Input: part model. Units: mm. Frame: model coordinates. Round coordinates to 2 decimals unless told otherwise and drop trailing zeros. Write each question's results on one line, items separated by ' | '.
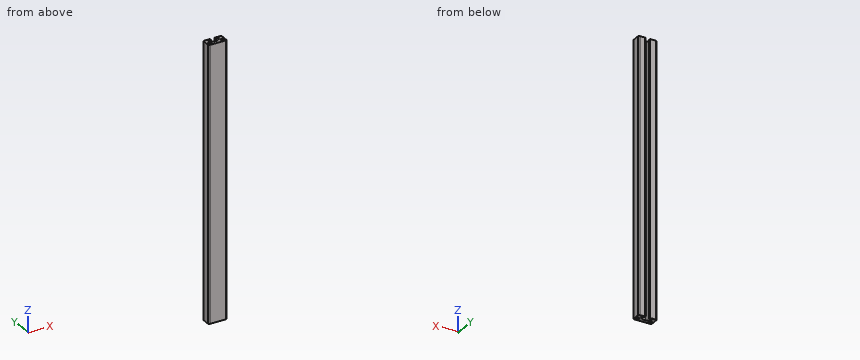
from build123d import *

# Parameters (mm, degrees)
SKETCH3_R           = 2.1463
BOSS_EXTRUDE1_DEPTH = 190.5
FILLET1_R           = 0.254


with BuildPart() as part:
    # Sketch3 → Boss-Extrude1 (new body, symmetric)
    with BuildSketch(Plane.XY):
        with BuildLine():
            Line((-11.049, 12.7), (-3.302, 12.7))
            Line((-3.302, 12.7), (-3.302, 10.328863887))
            Line((-3.302, 10.328863887), (-6.985, 10.328863887))
            ThreePointArc((-6.985, 10.328863887), (-7.454330803, 10.01526707), (-7.344210245, 9.461653642))
            Line((-7.344210245, 9.461653642), (-3.452505379, 5.569948776))
            ThreePointArc((-3.452505379, 5.569948776), (-2.628470073, 5.019345987), (-1.656454155, 4.826))
            Line((-1.656454155, 4.826), (1.656454155, 4.826))
            ThreePointArc((1.656454155, 4.826), (2.628470073, 5.019345987), (3.452505379, 5.569948776))
            Line((3.452505379, 5.569948776), (7.344210245, 9.461653642))
            ThreePointArc((7.344210245, 9.461653642), (7.454330803, 10.01526707), (6.985, 10.328863887))
            Line((6.985, 10.328863887), (3.302, 10.328863887))
            Line((3.302, 10.328863887), (3.302, 12.7))
            Line((3.302, 12.7), (11.049, 12.7))
            ThreePointArc((11.049, 12.7), (12.216433296, 12.216433296), (12.7, 11.049))
            Line((12.7, 11.049), (12.7, 1.651))
            ThreePointArc((12.7, 1.651), (12.216433296, 0.483566704), (11.049, 0))
            Line((11.049, 0), (-11.049, 0))
            ThreePointArc((-11.049, 0), (-12.216433296, 0.483566704), (-12.7, 1.651))
            Line((-12.7, 1.651), (-12.7, 11.049))
            ThreePointArc((-12.7, 11.049), (-12.216433296, 12.216433296), (-11.049, 12.7))
        make_face()
        with Locations((8.509, 4.064)):
            Circle(SKETCH3_R, mode=Mode.SUBTRACT)
        with Locations((-8.509, 4.064)):
            Circle(SKETCH3_R, mode=Mode.SUBTRACT)
    extrude(amount=BOSS_EXTRUDE1_DEPTH, both=True)

    # Fillet1
    fillet1_edges = [part.edges().sort_by_distance(p)[0] for p in [
        (-3.302, 12.7, 0),
        (-3.302, 10.328863887, 0),
        (3.302, 10.328863887, 0),
        (3.302, 12.7, 0),
    ]]
    fillet(fillet1_edges, radius=FILLET1_R)


solid = part.part
1. Section query A-A, the plane z = 158.5. Count the separate pieces of the cut face and the enclosed holes in it, plus the area to 3 significant figures.
Answer:
separate pieces: 1 | enclosed holes: 2 | area: 216 mm^2
2. Contact query for a flat-ended pin moving along its axis: pin 1 (3.5 mm diameter, centred on x = -0.5, z = -2.5, fed in from +Y). Output: stop coordinate, or through.
Answer:
pin 1: y = 4.9
3. Line query: line 1 (X direction, y = 11, z = 91); line 2 (Y direction, x = 3.5, z = -4); line 3 (X direction, y = 11.5, z = -140). Output: solid intervals per line, ascending. Write a range as [from, to].
Answer:
line 1: [-12.7, -3.3], [3.3, 12.7] | line 2: [0, 5.62], [10.34, 12.69] | line 3: [-12.64, -3.3], [3.3, 12.64]
